from build123d import *

# Parameters (mm, degrees)
SKETCH_1_W          = 64.494727868
SKETCH_1_H          = 65
SKETCH_1_R          = 1.65
EXTRUDE_1_DEPTH     = 10
SKETCH_2_R          = 1.65
CUT_EXTRUDE_1_DEPTH = 47.863018263
SKETCH_3_R          = 1.65
CUT_EXTRUDE_2_DEPTH = 44.110090197
FILLET_1_R          = 6


with BuildPart() as part:
    # ｽｹｯﾁ1 → ﾎﾞｽ - 押し出し1 (new body)
    with BuildSketch(Plane(origin=(0, 0, 0), x_dir=(0, 0, -1), z_dir=(1, 0, 0))):
        Rectangle(SKETCH_1_W, SKETCH_1_H)
        Circle(SKETCH_1_R, mode=Mode.SUBTRACT)
        with Locations((-9.255829981, -23.223471131)):
            Circle(SKETCH_1_R, mode=Mode.SUBTRACT)
        with Locations((-22.247363934, -11.404157049)):
            Circle(SKETCH_1_R, mode=Mode.SUBTRACT)
    extrude(amount=EXTRUDE_1_DEPTH)

    # ｽｹｯﾁ2 → ｶｯﾄ - 押し出し1 (cut, through all)
    with BuildSketch(Plane(origin=(10, 0, 0), x_dir=(0, 0, -1), z_dir=(1, 0, 0))):
        with BuildLine():
            Line((9.743790334, 32.5), (9.743790334, 4.190292345))
            Line((9.743790334, 4.190292345), (-2.288788642, -26.000220125))
            ThreePointArc((-2.288788642, -26.000220125), (-12.032578975, -30.19051247), (-16.22287132, -20.446722136))
            Line((-16.22287132, -20.446722136), (-5.256209666, 7.069335401))
            Line((-5.256209666, 7.069335401), (-5.256209666, 32.5))
            Line((-5.256209666, 32.5), (-32.247363934, 32.5))
            Line((-32.247363934, 32.5), (-32.247363934, -32.5))
            Line((-32.247363934, -32.5), (32.247363934, -32.5))
            Line((32.247363934, -32.5), (32.247363934, 32.5))
            Line((32.247363934, 32.5), (9.743790334, 32.5))
        make_face()
        with Locations((-22.247363934, -11.404157049)):
            Circle(SKETCH_2_R, mode=Mode.SUBTRACT)
    extrude(amount=-CUT_EXTRUDE_1_DEPTH, mode=Mode.SUBTRACT)

    # ｽｹｯﾁ3 → ｶｯﾄ - 押し出し2 (cut, through all)
    with BuildSketch(Plane(origin=(0, 0, -9.743790334), x_dir=(-1, 0, 0), z_dir=(0, 0, -1))):
        with Locations(Location((-5, 27.5, 0), (0, 0, 90))):
            Circle(SKETCH_3_R)
        with Locations(Location((-5, 17.5, 0), (0, 0, 90))):
            Circle(SKETCH_3_R)
    extrude(amount=-CUT_EXTRUDE_2_DEPTH, mode=Mode.SUBTRACT)

    # ﾌｨﾚｯﾄ1
    fillet_1_edges = [part.edges().sort_by_distance(p)[0] for p in [
        (5, 7.069335401, 5.256209666),
        (5, 4.190292345, -9.743790334),
    ]]
    fillet(fillet_1_edges, radius=FILLET_1_R)


solid = part.part
Verification items for the finished model (mm, model axes). A direction names the side the tool comes from. Coordinates: 2 decimals unless noted, no trailing zeros. Order: outer loops, then holes, each group sorted by start corner. A loop starts at its lowest first (then second) coordinate and runs counter-clockwise, first axis right, second up.
Item 1: Material ranges on L1, parallel to X at y = 27.5, z = -4.5; L2, parallel to Y at x = 6.5, z = 3; L3, parallel to Z at x = 3.75, y = -24, recorded low to high.
Filled in:
L1: x = 0 to 3.35, 6.65 to 10
L2: y = -27.36 to 16.81, 18.19 to 26.81, 28.19 to 32.5
L3: z = 1.49 to 7.8, 10.71 to 16.72
Item 2: Release check for a two-part mould opening along Y. For faces 3 (the face through (5, 32.5, -2)), 4 (the face through (4.93, 1.115, 1.216)), 5 (the face through (0, 1, 4)) record: +Y half, -Y half, draft (parallel to the pull), parting line (faces both ways), or undercut.
Filled in:
face 3: +Y half
face 4: undercut
face 5: draft
Item 3: Section check C-C, the plane x = 5.75. Enter the section's corners in (y, z).
Filled in:
outline: (-26, 2.29) - (3.12, -9.32) arc R6 ccw to (5.34, -9.74) - (16.03, -9.74) - (16.03, 5.26) - (8.22, 5.26) arc R6 cw to (6, 5.68) - (-20.45, 16.22) arc R7.5 ccw to start; (18.97, -9.74) - (26.03, -9.74) - (26.03, 5.26) - (18.97, 5.26) - close; (28.97, -9.74) - (32.5, -9.74) - (32.5, 5.26) - (28.97, 5.26) - close; hole circle Ø3.3 at (-23.22, 9.26); hole circle Ø3.3 at (0, 0)
Item 4: Depth check by flat-ended pin: pin 1 (4.5 mm diameter, centred on x = 5, y = 27.5, fed in from -Z); pin 2 (5 mm diameter, centred on x = 6, y = -20.5, fed in from +Z). Enter the tip coordinate at first touch or a pass-through.
Filled in:
pin 1: stops at z = -9.74
pin 2: stops at z = 16.75
Item 5: Access from +Z, -Z, +X, -X, +Y, -Y to the whole of each face (thin tool, end or side, straight path). Record for faces 1 (the face through (4.93, 4.23, -9.64)), 2 (the face through (5, 20, 5.256)).
Filled in:
face 1: -Z, +X, -X, -Y
face 2: +Z, +X, -X, +Y
Item 6: Section check A-A, the plane z = 0. Enter the section's corners in (x, y).
Filled in:
outline: (0, -20.26) - (10, -20.26) - (10, -1.65) - (0, -1.65) - close; (0, 1.65) - (10, 1.65) - (10, 32.5) - (0, 32.5) - close; hole circle Ø3.3 at (5, 17.5); hole circle Ø3.3 at (5, 27.5)
Item 7: Section check B-B, the plane y = 17.5. Enter the section's corners in (x, z), then the cut area to 4 significant figures.
Filled in:
outline: (0, -9.74) - (3.35, -9.74) - (3.35, 5.26) - (0, 5.26) - close; (6.65, -9.74) - (10, -9.74) - (10, 5.26) - (6.65, 5.26) - close
area: 100.5 mm2
Item 8: Section check D-D, the plane x = 1. Enter the section's corners in (y, z), then the cut area to 3 significant figures.
Filled in:
outline: (-26, 2.29) - (3.12, -9.32) arc R6 ccw to (5.34, -9.74) - (32.5, -9.74) - (32.5, 5.26) - (8.22, 5.26) arc R6 cw to (6, 5.68) - (-20.45, 16.22) arc R7.5 ccw to start; hole circle Ø3.3 at (-23.22, 9.26); hole circle Ø3.3 at (0, 0)
area: 940 mm2
